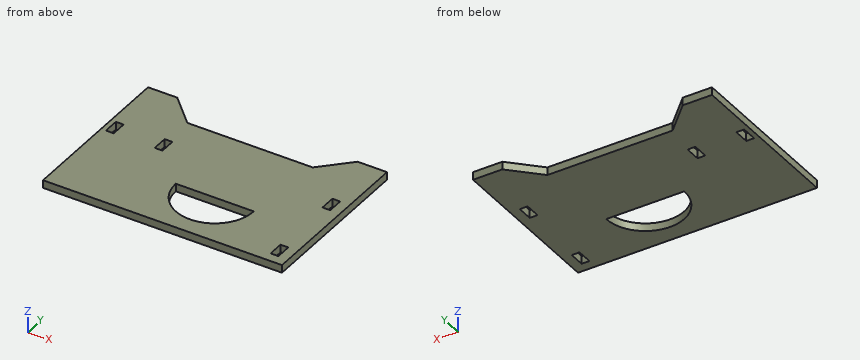
from build123d import *

# Parameters (mm, degrees)
SKETCH1_W           = 122.5
SKETCH1_H           = 60
SKETCH1_W_2         = 4
SKETCH1_H_2         = 8
BOSS_EXTRUDE1_DEPTH = 4
BOSS_EXTRUDE2_DEPTH = 4


with BuildPart() as part:
    # Sketch1 → Boss-Extrude1 (new body)
    with BuildSketch(Plane.XY):
        with Locations((-8.75, 0)):
            Rectangle(SKETCH1_W, SKETCH1_H)
        with BuildLine():
            Line((-20, -1.498357325), (20, -1.498357325))
            ThreePointArc((20, -1.498357325), (0, -21.498357325), (-20, -1.498357325))
        make_face(mode=Mode.SUBTRACT)
        with Locations((-40.5, 21)):
            Rectangle(SKETCH1_W_2, SKETCH1_H_2, mode=Mode.SUBTRACT)
        with Locations((45.5, 21)):
            Rectangle(SKETCH1_W_2, SKETCH1_H_2, mode=Mode.SUBTRACT)
        with Locations((45.5, -21)):
            Rectangle(SKETCH1_W_2, SKETCH1_H_2, mode=Mode.SUBTRACT)
        with Locations((-65.5, 21)):
            Rectangle(SKETCH1_W_2, SKETCH1_H_2, mode=Mode.SUBTRACT)
    extrude(amount=BOSS_EXTRUDE1_DEPTH)

    # Sketch2 → Boss-Extrude2 (add)
    with BuildSketch(Plane.XY):
        Polygon((-70, 30), (52.5, 30), (52.5, 55), (37.5, 55), (23.357864376, 40.857864376), (-40.857864376, 40.857864376), (-55, 55), (-70, 55), align=None)
    extrude(amount=BOSS_EXTRUDE2_DEPTH)


solid = part.part
Can you work these out from the model? Positions are in its coordinate system, mm. Coordinates: 2 decimals unless noted, no trailing zeros. Write each loop counter-clockwise with the first axis right and the second up, starting at its lowest first coordinate (ties: lowest second). Pieces come first, ordered by that corner, then holes. Notation, with made-up numbers: (-5, 14) -> (5, 14) arc R12 ccw to (5, 28) -> close; hole circle Ø2 at (-7, 51.5). An arc over 180 degrees is marked (long way). Write each question's results on one line, items separated by ' | '. Start each with the question number.
Q1. Imagine slicing it at B-B (x = 0). Write out the boundary of the cut face in (y, z), then the cut area to 3 significant figures.
Q2. If I drill on probe 1 along Y at (x, z) = (-1, 3.05); probe 2 along Y at (x, z) = (-33, 2.75); probe 3 along X at (y, z) = (-5.5, 0.25), over which ranges is the centre line in solid material (lowest first)?
Q3. Imagine slicing it at A-A (y = 19). Write out the boundary of the cut face in (x, z).
Q4. Imagine slicing it at D-D (y = -7.5). Write out the boundary of the cut face in (x, z), then the cut area to 3 significant figures.
Q5. Imagine slicing it at C-C (z = 0.85). Write out the boundary of the cut face in (x, y), then the cut area to 3 significant figures.
Taken from the geometry:
1) outline: (-30, 0) -> (-21.5, 0) -> (-21.5, 4) -> (-30, 4) -> close; (-1.5, 0) -> (40.86, 0) -> (40.86, 4) -> (-1.5, 4) -> close | area: 203 mm^2
2) probe 1: y = -30 to -21.47, -1.5 to 40.86 | probe 2: y = -30 to 40.86 | probe 3: x = -70 to -19.6, 19.6 to 52.5
3) outline: (-70, 0) -> (-67.5, 0) -> (-67.5, 4) -> (-70, 4) -> close; (-63.5, 0) -> (-42.5, 0) -> (-42.5, 4) -> (-63.5, 4) -> close; (-38.5, 0) -> (43.5, 0) -> (43.5, 4) -> (-38.5, 4) -> close; (47.5, 0) -> (52.5, 0) -> (52.5, 4) -> (47.5, 4) -> close
4) outline: (-70, 0) -> (-19.08, 0) -> (-19.08, 4) -> (-70, 4) -> close; (19.08, 0) -> (52.5, 0) -> (52.5, 4) -> (19.08, 4) -> close | area: 337 mm^2
5) outline: (-70, -30) -> (52.5, -30) -> (52.5, 55) -> (37.5, 55) -> (23.36, 40.86) -> (-40.86, 40.86) -> (-55, 55) -> (-70, 55) -> close; hole (-67.5, 17) -> (-63.5, 17) -> (-63.5, 25) -> (-67.5, 25) -> close; hole (-42.5, 17) -> (-38.5, 17) -> (-38.5, 25) -> (-42.5, 25) -> close; hole (-20, -1.5) arc R20 ccw to (20, -1.5) -> close; hole (43.5, -25) -> (47.5, -25) -> (47.5, -17) -> (43.5, -17) -> close; hole (43.5, 17) -> (47.5, 17) -> (47.5, 25) -> (43.5, 25) -> close | area: 8,550 mm^2
